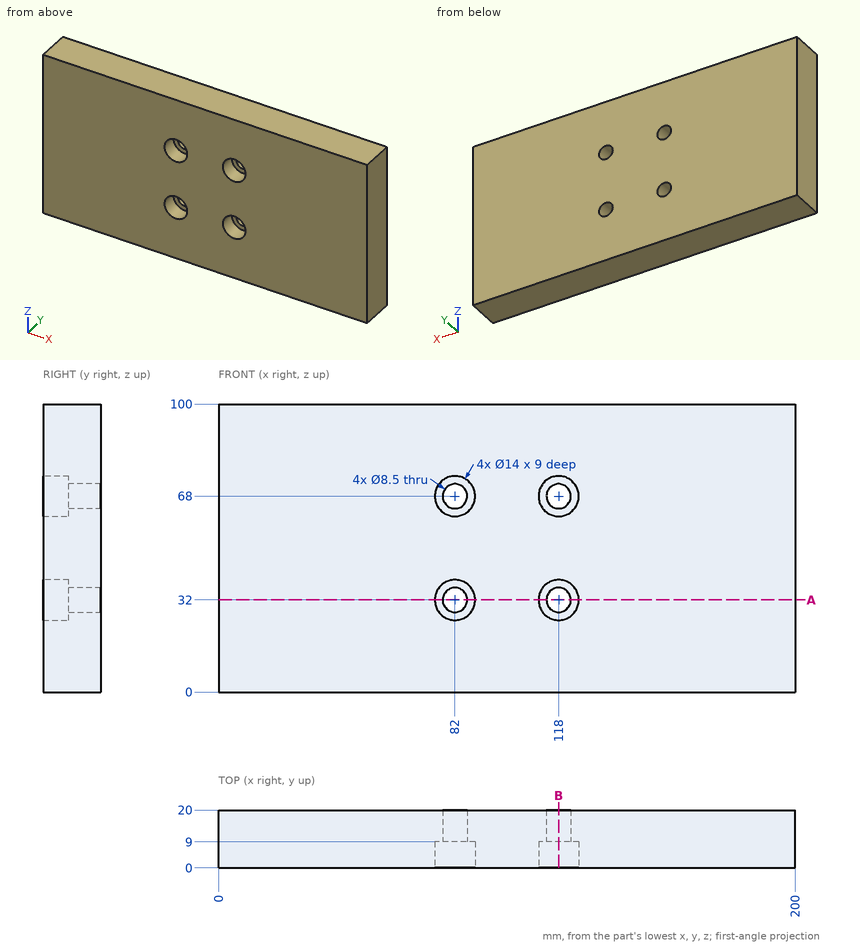
Here's the drawing with two shaded views (mm, measured from the low corner). I have some questions. Coordinates: 2 decimals unless noted, no trailing zeros. Order: outer loops, then holes, each group sorted by start corner. A loop starts at its lowest first (then second) coordinate and runs counter-clockwise, first axis right, second up. Notation, with made-up numbers: M -9.75,48 L 9.25,48 A12 ccw 9.25,53 Z; hole C 21.5,56 d5. An arc over 180 degrees is marked long. Answer as CSV lines item,"result".
Item 1: Imagine slicing it at A-A on z = 32. Write out the boundary of the cut face in (x, y), plus the area to 3 significant figures.
Results found:
outline,"M 0,0 L 75,0 L 75,9 L 77.75,9 L 77.75,20 L 0,20 Z; M 86.25,9 L 89,9 L 89,0 L 111,0 L 111,9 L 113.75,9 L 113.75,20 L 86.25,20 Z; M 122.25,9 L 125,9 L 125,0 L 200,0 L 200,20 L 122.25,20 Z"
area,"3,560 mm2"
Item 2: If I drill on line 1 (X direction, y = 3.75, z = 68); line 2 (Z direction, x = 112, y = 1.5); line 3 (X direction, y = 13.75, z = 68), over which ranges is the centre line in solid material (lowest first)?
Results found:
line 1,"0 to 75, 89 to 111, 125 to 200"
line 2,"0 to 28.39, 35.61 to 64.39, 71.61 to 100"
line 3,"0 to 77.75, 86.25 to 113.75, 122.25 to 200"
Item 3: Imagine slicing it at B-B on x = 118. Write out the boundary of the cut face in (y, z).
Results found:
outline,"M 0,0 L 20,0 L 20,27.75 L 9,27.75 L 9,25 L 0,25 Z; M 0,39 L 9,39 L 9,36.25 L 20,36.25 L 20,63.75 L 9,63.75 L 9,61 L 0,61 Z; M 0,75 L 9,75 L 9,72.25 L 20,72.25 L 20,100 L 0,100 Z"
Item 4: For pin 1 (10 mm diameter, centred on x = 82, z = 68, fed in from -Y), with a flat end and sliding along its axis, tell me the tip position at first contact or that it passes through.
Results found:
pin 1,"y = 9"
